Geometry check sheet. Reference: the model listing, model coordinates, mm. Face numbers are marked on the shaded views. A direction names the side the tool comes from. Give positions to 0.01 mm unless a question says otherwise; leave off trailing zeros. Loops run counter-clockwise (first coordinate to the right, second up) from the corner with the lowest first, then second, coordinate; pieces in that order, holes last. Notation, with made-up numbers: (85.5, 77.25) -> (138.5, 77.25) arc R13 cw to (138.5, 90.25) -> close; hole circle Ø4 at (60, 36). An arc over 180 degrees is marked (long way). Write each question's results on one line, items separated by ' | '. Start each with the question number.
1) Draft check along Y on the marked faces 1, 2 and 3. Enter one of: pulls with the +Y half, pulls with the -Y half, needs draft (parallel to the pull), parting line crosses it, or undercut.
2) Sectioned sample at A-A on z = 0. Record the cut outline in (x, y).
3) Sectioned sample at D-D on y = 3.75. Record the cut outline in (x, z).
4) Sectioned sample at C-C on z = 5.5. Record the cut outline in (x, y).
5) Scan lines: line 1 (X direction, y = 1.75, z = 0); line 2 (Y direction, x = 0, z = 4.4); line 3 (Y direction, x = 0, z = 5.85). Record each from-to range of solid material in increasing order. Write a range as from..to.
6) Depth check by flat-ended pin: pin 1 (3 mm diameter, centred on x = 0, y = 4.95, fed in from +Z); pin 2 (4 mm diameter, centred on y = 6, z = 4, fed in from +X); pin 3 (7 mm diameter, centred on x = 0, z = 0, fed in from -Y); pin 4 (1.8 mm diameter, centred on x = 0, y = 5.02, fed in from -Z). Enter the tip coordinate at first touch or a pass-through.
7) Sectioned sample at B-B on x = 3.25. Record the cut outline in (y, z), then the cut area to 3 significant figures.
8) Set-up check for the marked faces 4 and 5: record each of +Z, -Z, +X, -X, +Y, -Y from which the full face is reachable in a straight line by a thin tool's end or side.
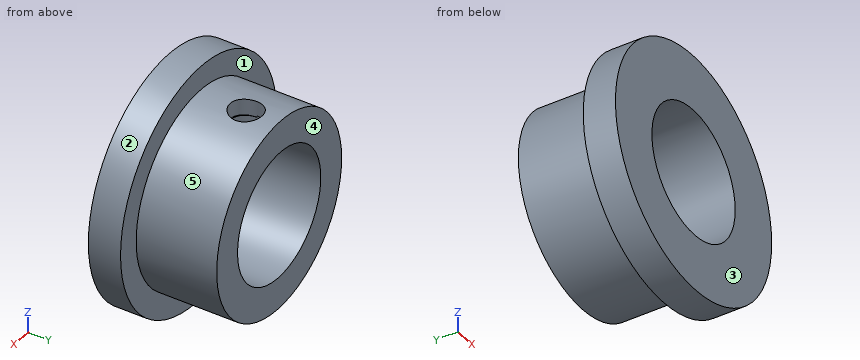
Autodesk Fusion 360 part; units mm, degrees
sketch "Sketch1" plane through (0, 0, 0) normal (0, 1, 0) x (1, 0, 0)
  circle A0 centre (0, 0) radius 5
  circle A1 centre (0, 0) radius 7.5
  dimension "d1" = 15
extrude "Extrude1" add sketch "Sketch1" along normal blind 2
sketch "Sketch2" plane through (0, 2, 0) normal (0, 1, 0) x (-1, 0, 0)
  circle A0 centre (0, 0) radius 5
  circle A1 centre (0, 0) radius 7.5
  circle A2 centre (0, 0) radius 6
extrude "Extrude2" add sketch "Sketch2" along normal blind 5 contours A2
hole "Hole1" at (0, 4.9495, 6) direction (0, 0, -1) diameter 2 depth 6 tip angle 118
sketch "Sketch3" plane through (0, 0, 0) normal (0, 1, 0) x (1, 0, 0)
  circle A0 centre (0, 0) radius 4
  circle A1 centre (0, 0) radius 5
extrude "Extrude3" add sketch "Sketch3" along normal blind 7
hole "Hole2" at (0, 5.0219, 5) direction (0, 0, -1) diameter 2 depth 1 tip angle 118
Result:
1) face 1: pulls with the +Y half | face 2: needs draft | face 3: pulls with the -Y half
2) outline: (-7.5, 0) -> (-4, 0) -> (-4, 7) -> (-6, 7) -> (-6, 2) -> (-7.5, 2) -> close; (4, 0) -> (7.5, 0) -> (7.5, 2) -> (6, 2) -> (6, 7) -> (4, 7) -> close
3) outline: circle Ø12 at (0, 0); hole circle Ø8 at (0, 0)
4) outline: (-5.1, 0) -> (5.1, 0) -> (5.1, 2) -> (2.4, 2) -> (2.4, 7) -> (-2.4, 7) -> (-2.4, 2) -> (-5.1, 2) -> close; hole circle Ø2 at (0, 4.95)
5) line 1: -7.5..-4, 4..7.5 | line 2: 0..4.02, 6.02..7 | line 3: 0..3.95, 5.95..7
6) pin 1: z = 6 | pin 2: x = 5.66 | pin 3: through | pin 4: z = -6
7) outline: (0, -6.76) -> (2, -6.76) -> (2, -5.04) -> (7, -5.04) -> (7, -2.33) -> (0, -2.33) -> close; (0, 2.33) -> (7, 2.33) -> (7, 5.04) -> (2, 5.04) -> (2, 6.76) -> (0, 6.76) -> close | area: 44.8 mm^2
8) face 4: +Z, -Z, +X, -X, +Y | face 5: +Y
